Here's the drawing with two shaded views (mm, measured from the low corner). I have some questions. A direction names the side the tool comes from. Coordinates: 2 decimals unless noted, no trailing zeros. Loops run counter-clockwise (first coordinate to the right, second up) from the corner with the lowest first, then second, coordinate; pieces in that order, holes last. Notation, with made-up numbers: (60, 39) -> (68, 39) arc R7 ccw to (68, 52) -> close; hole circle Ø5 at (9, 39). An arc over 180 degrees is marked (long way). Answer as a JSON object with one key per item and string values. Group by question number.
1) I want a section at C-C (x = 88.5). Write out the boundary of the cut face in (y, z), then the cut area to 3 significant figures.
2) I want a section at D-D (y = 58). Write out the boundary of the cut face in (x, z), then the cut area to 3 significant figures.
3) I want a section at B-B (z = 113). Write out the boundary of the cut face in (x, y), then the cut area to 3 significant figures.
4) I'm going to push flat-ended pins straight in: pin 1 (19 mm diameter, centred on x = 101.5, y = 28.5, fed in from -Z); pin 2 (7.5 mm diameter, centred on x = 75, z = 166, fed in from -Y); pin 3 (12 mm diameter, centred on x = 91, z = 79.5, fed in from +Y). Where does each tip first touch, or does it pass through?
5) I need wall thicknesses on probe 1 along X at (y, z) = (34, 88); probe 2 along Y at (x, z) = (110, 89); probe 3 along Y at (x, z) = (70.5, 168). Which ranges of each line are inside material? Lowest first, please. Write a range as [from, to].
6) Which directions (+Z, -Z, +X, -X, +Y, -Y) give clear straight access to the entire face, cutting with the end or side of a thin tool? Please do the marked faces 1, 2, 3, 4 and 5.
7) I want a section at A-A (y = 90). Write out the boundary of the cut face in (x, z).
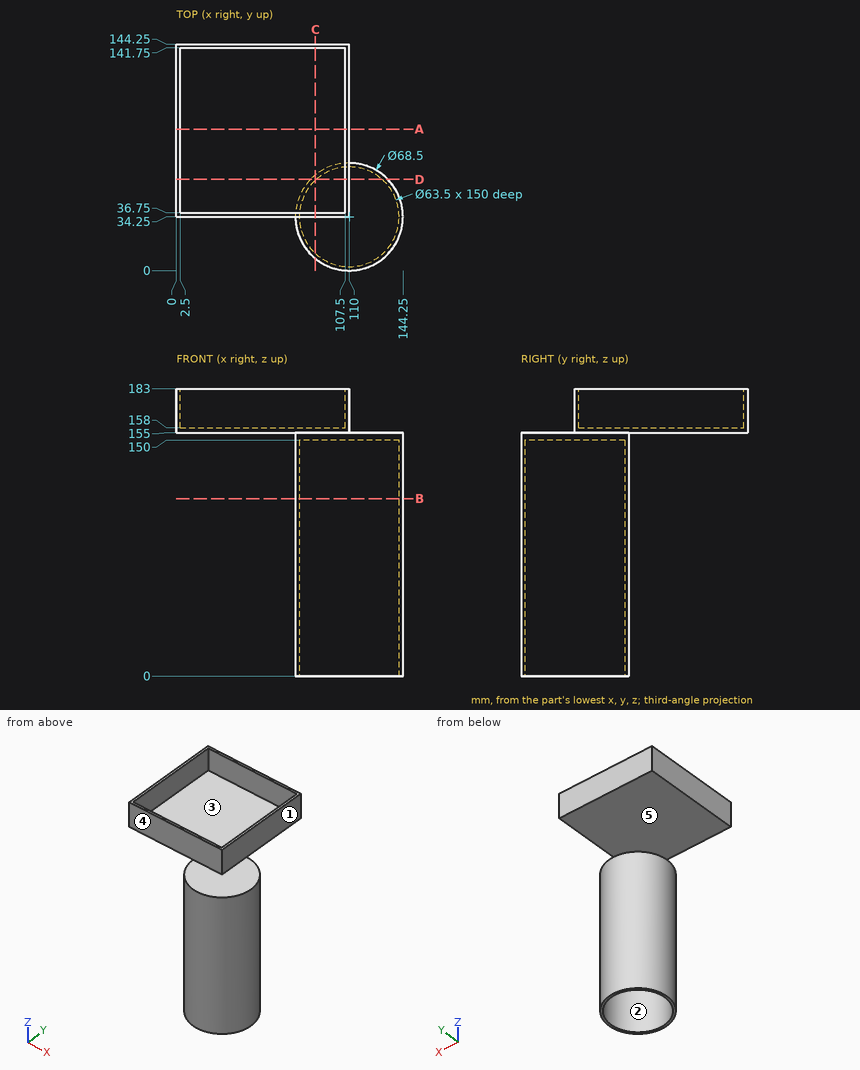
Determined:
{
 "1": {"outline": "(7.59, 0) -> (10.89, 0) -> (10.89, 150) -> (57.61, 150) -> (57.61, 0) -> (60.91, 0) -> (60.91, 155) -> (144.25, 155) -> (144.25, 183) -> (141.75, 183) -> (141.75, 158) -> (36.75, 158) -> (36.75, 183) -> (34.25, 183) -> (34.25, 155) -> (7.59, 155) -> close", "area": "1,710 mm^2"},
 "2": {"outline": "(0, 155) -> (85.32, 155) -> (85.32, 0) -> (88.93, 0) -> (88.93, 150) -> (131.07, 150) -> (131.07, 0) -> (134.68, 0) -> (134.68, 155) -> (110, 155) -> (110, 183) -> (107.5, 183) -> (107.5, 158) -> (2.5, 158) -> (2.5, 183) -> (0, 183) -> close", "area": "1,780 mm^2"},
 "3": {"outline": "circle Ø68.5 at (110, 34.25); hole circle Ø63.5 at (110, 34.25)", "area": "518 mm^2"},
 "4": {"pin 1": "z = 150", "pin 2": "y = 34.25", "pin 3": "y = 65.94"},
 "5": {"probe 1": "[75.75, 78.25], [141.75, 144.25]", "probe 2": "[0, 2.5], [66, 68.5]", "probe 3": "[34.25, 36.75], [141.75, 144.25]"},
 "6": {"face 1": "+Z, +X, +Y, -Y", "face 2": "-Z", "face 3": "+Z", "face 4": "+Z, +X, -X, -Y", "face 5": "-Z, -X, +Y"},
 "7": {"outline": "(0, 155) -> (110, 155) -> (110, 183) -> (107.5, 183) -> (107.5, 158) -> (2.5, 158) -> (2.5, 183) -> (0, 183) -> close"}
}
